Could you check a few things on this drawing? It's one solid part, dimensions in mm from its lowest x, y, z. A direction names the side the tool comes from. Give positions to 0.01 mm unless a question says otherwise; leave off trailing zeros. Order: outer loops, then holes, each group sorted by start corner. A loop starts at its lowest first (then second) coordinate and runs counter-clockwise, first axis right, second up.
(1) Imagine slicing it at A-A, the plane y = 9. Write out the boundary of the cut face in (x, z).
(2) If I drill on probe 1 along Y at (x, z) = (57, 15.5); probe 2 along Y at (x, z) = (8.5, 15); probe 3 along Z at (x, y) = (34.5, 5.5), over which ranges is the centre line in solid material (lowest first)?
(3) On a 3-axis mill with a long thin cutter (end or side, diameter ignored), from which of +Z, -Z, +X, -X, +Y, -Y can I reach the whole of each face in a straight line? I mean the marked faces 1 and 2. Say none if no direction works.
(4) If we mould it in two halves opening along Y, with no side actions, what happens to the marked faces 3 and 4? For each: released by +Y, released by -Y, zero draft, split by the parting line, or undercut.
(5) Imagine slicing it at C-C, the plane x = 29.5. Write out the boundary of the cut face in (y, z).
(6) Will these pins go through, and if not, where does the flat tip stop? pin 1 (4 mm diameter, centred on x = 26.5, y = 4, fed in from -Z); pin 2 (5 mm diameter, centred on x = 14, y = 12, fed in from -Z); pin 3 (1.5 mm diameter, centred on x = 27.5, z = 5, fed in from +Y).
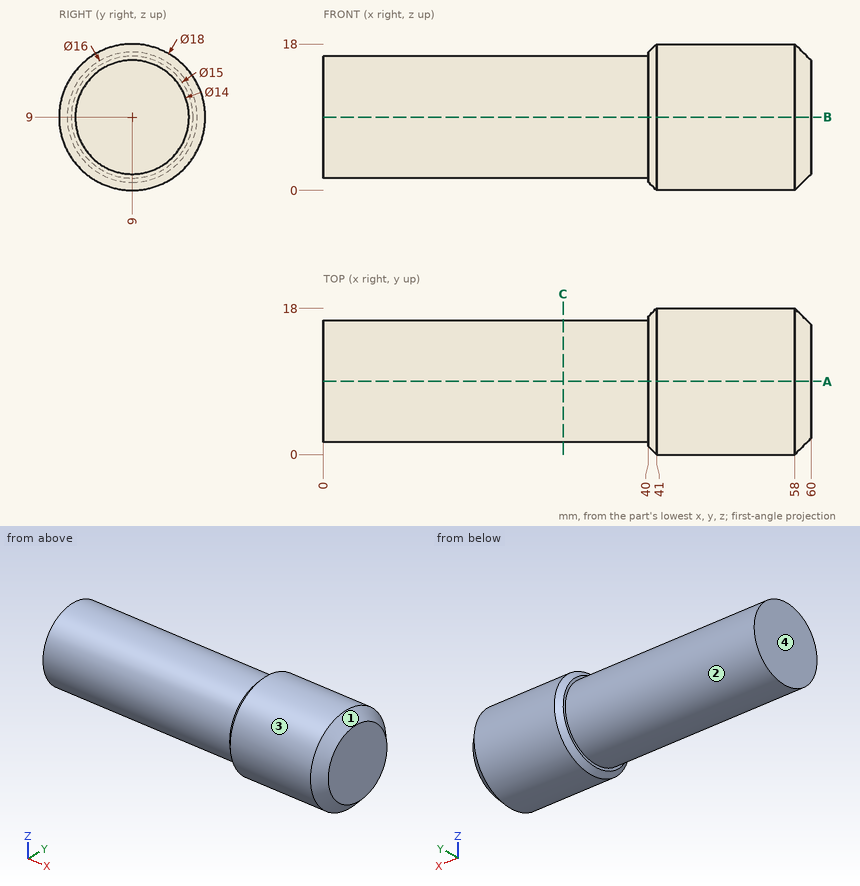
Answer block:
1. outline: (0, 1.5) - (40, 1.5) - (40, 1) - (41, 0) - (58, 0) - (60, 2) - (60, 16) - (58, 18) - (41, 18) - (40, 17) - (40, 16.5) - (0, 16.5) - close
2. probe 1: y = 2.78 to 15.22
2. probe 2: y = 4.5 to 13.5
2. probe 3: z = 2.37 to 15.63
3. face 1: +X
3. face 2: -X
4. face 3: split by the parting line
4. face 4: zero draft
5. outline: circle Ø15 at (9, 9)
6. pin 1: stops at z = 2.13
6. pin 2: stops at z = 1.52
6. pin 3: stops at y = 15.76
